from build123d import *

# Parameters (mm, degrees)
F0_R     = 9.525
F0_R_2   = 7.8105
F0_R_3   = 6.096
F0_R_4   = 4.826
F0_R_5   = 1.905
F1_DEPTH = 2.032
F2_DEPTH = 9.525
F3_R     = 4.7625
F4_DEPTH = 3.175


with BuildPart() as f1:
    # F0 (on Top) → F1 (new body)
    with BuildSketch(Plane.XY):
        Circle(F0_R)
        Circle(F0_R_2, mode=Mode.SUBTRACT)
        Circle(F0_R_2)
        Circle(F0_R_3, mode=Mode.SUBTRACT)
        Circle(F0_R_3)
        Circle(F0_R_4, mode=Mode.SUBTRACT)
        Circle(F0_R_4)
        Circle(F0_R_5, mode=Mode.SUBTRACT)
    extrude(amount=-F1_DEPTH)

    # F0 (on Top) → F2 (join)
    with BuildSketch(Plane.XY):
        Circle(F0_R)
        Circle(F0_R_2, mode=Mode.SUBTRACT)
    extrude(amount=F2_DEPTH)

    # F3
    f3_edges = [f1.edges().sort_by_distance(p)[0] for p in [
        (-9.525, 0, -2.032),
    ]]
    fillet(f3_edges, radius=F3_R)

    # F0 (on Top) → F4 (join)
    with BuildSketch(Plane.XY):
        Circle(F0_R_4)
        Circle(F0_R_5, mode=Mode.SUBTRACT)
    extrude(amount=F4_DEPTH)


solid = f1.part
Read the model definition and answer for the solid it produces. Units are mm, in the model's axes. A direction names the side the tool comes from. Round coordinates to 2 decimals unless told otherwise and drop trailing zeros.
Q1. Which of the six approach directions +Z, -Z, +X, -X, +Y, -Y give full straight-line access (tool end or side, diameter ignored) to faces 5 (the face through (-3.83, -2.937, 1.565)), 6 (the face through (-2.2, 0.1, -2.032))?
Q2. Each of these flat-tipped pins is pushed along its axis until it touches: pin 1 (6 mm diameter, centred on x = 0, y = 0, fed in from +Z) (3 decimals); pin 2 (1 mm diameter, centred on x = 0.5, z = 3.5, fed in from -Y) (3 decimals); pin 3 (3 mm diameter, centred on x = 4.5, z = 5.5, fed in from +Y); pin 4 (1 mm diameter, centred on x = 2.5, z = 8, fed in from -Y). Where does it stop, or does it pass through?
Q3. Determine the mould class of faces 1 (the face through (3, 4, 0)), 2 (the face through (-1.017, 7.744, 4.696)), 3 (the face through (-1, 8, 9.525)), 4 (the face through (-7.559, -5.796, 6.08)) for opening direction Y: released by +Y, released by -Y, zero draft, split by the parting line, or undercut.
Q4. Consider probe 1 along Y at (x, z) = (0, 2.75) (1 decimal); probe 2 along X at (y, z) = (3.75, 3); probe 3 along Y at (x, z) = (0.5, 1). Determine where each line is inside the solid, lowest interval first.
Output:
1. face 5: +Z
1. face 6: -Z, +X, -X, +Y, -Y
2. pin 1: stops at z = 3.175
2. pin 2: stops at y = -9.525
2. pin 3: stops at y = 9.04
2. pin 4: stops at y = -9.31
3. face 1: undercut
3. face 2: undercut
3. face 3: zero draft
3. face 4: split by the parting line
4. probe 1: y = -9.5 to -7.8, -4.8 to -1.9, 1.9 to 4.8, 7.8 to 9.5
4. probe 2: x = -8.76 to -6.85, -3.04 to 3.04, 6.85 to 8.76
4. probe 3: y = -9.19 to -7.79, -4.8 to -1.84, 1.84 to 4.8, 7.79 to 9.19
